For this review, take the finished solid that the model builds, in its own axes (mm). Give positions to 0.01 mm unless a question says otherwise; leave off trailing zeros. Write each loop counter-clockwise with the first axis right and the second up, starting at its lowest first coordinate (ties: lowest second). Pieces come first, ordered by that corner, then holes.
1) We need section A-A on x = 68. Give the boundary of the cut face in (y, z).
2) We need section C-C on x = 9. Give the boundary of the cut face in (y, z), and give its area (3 significant figures).
3) Wall thickness on line 1 along Y through (x, z) = (111, -2.2); line 2 along Y through (x, z) = (90, -2); line 3 along Y through (x, z) = (56, -2): over which ranges is each line inside the solid? List them lowest first.
4) For P1, Ø5, axis at x = 30, y = 98, coming from the -Z side, flat-tipped, find the tip position at first contact; note if it passes through.
5) We need section B-B on y = 22. Give the boundary of the cut face in (x, z), and give its area (3 significant figures).
Autodesk Inventor part; units mm, degrees
ref_plane "YZ Plane" through (0, 0, 0) normal (1, 0, 0) x (0, 1, 0)
ref_plane "XZ Plane" through (0, 0, 0) normal (0, 1, 0) x (-1, 0, 0)
ref_plane "XY Plane" through (0, 0, 0) normal (0, 0, 1) x (1, 0, 0)
sketch "Náčrt2" plane through (0, 0, 0) normal (0, 0, 1) x (1, 0, 0)
  line L0 (0, 0) -> (120, 0)
  line L1 (120, 0) -> (120, 120)
  line L2 (120, 120) -> (0, 120)
  line L3 (0, 120) -> (0, 0)
  circle A0 centre (34.5442, 85.4558) radius 2.5
  circle A1 centre (85.4558, 85.4558) radius 2.5
  circle A2 centre (34.5442, 34.5442) radius 2.5
  circle A3 centre (85.4558, 34.5442) radius 2.5
  circle A4 centre (40.5, 111) radius 2
  circle A5 centre (79.5, 111) radius 2
  circle A6 centre (9, 79.5) radius 2
  circle A7 centre (9, 40.5) radius 2
  circle A8 centre (111, 79.5) radius 2
  circle A9 centre (111, 40.5) radius 2
  circle A10 centre (79.5, 9) radius 2
  circle A11 centre (40.5, 9) radius 2
  circle A12 centre (30, 98) radius 2
  circle A13 centre (90, 98) radius 2
  circle A14 centre (90, 22) radius 2
  circle A15 centre (30, 22) radius 2
  line L4 (42.5, 82.5) -> (77.5, 82.5)
  line L5 (82.5, 77.5) -> (82.5, 42.5)
  line L6 (77.5, 37.5) -> (42.5, 37.5)
  line L7 (37.5, 42.5) -> (37.5, 77.5)
  arc A16 (37.5, 42.5) -> (42.5, 37.5) centre (42.5, 42.5) ccw
  arc A17 (77.5, 37.5) -> (82.5, 42.5) centre (77.5, 42.5) ccw
  arc A18 (42.5, 82.5) -> (37.5, 77.5) centre (42.5, 77.5) ccw
  arc A19 (82.5, 77.5) -> (77.5, 82.5) centre (77.5, 77.5) ccw
  point P0 (37.5, 82.5)
  point P1 (82.5, 37.5)
  point P2 (82.5, 82.5)
  point P3 (37.5, 37.5)
  dimension "d18" = 1
  dimension "d26" = 120
  dimension "d27" = 120
  dimension "d28" = 39
  dimension "d29" = 39
  dimension "d30" = 60
  dimension "d31" = 76
  dimension "d32" = 72
  dimension "d35" = 5
  dimension "d36" = 4
  dimension "d37" = 4
  dimension "d42" = 5
  dimension "d43" = 5
  dimension "d44" = 35
extrude "Vysunutí2" add sketch "Náčrt2" against normal blind 3
properties part number "Cougar_Base2"
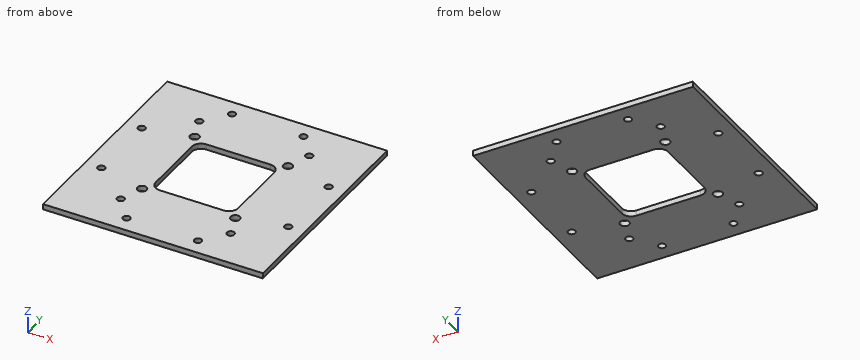
Results list:
1. outline: (0, -3) - (37.5, -3) - (37.5, 0) - (0, 0) - close; (82.5, -3) - (120, -3) - (120, 0) - (82.5, 0) - close
2. outline: (0, -3) - (38.5, -3) - (38.5, 0) - (0, 0) - close; (42.5, -3) - (77.5, -3) - (77.5, 0) - (42.5, 0) - close; (81.5, -3) - (120, -3) - (120, 0) - (81.5, 0) - close
2. area: 336 mm2
3. line 1: y = 0 to 38.5, 42.5 to 77.5, 81.5 to 120
3. line 2: y = 0 to 20, 24 to 96, 100 to 120
3. line 3: y = 0 to 37.5, 82.5 to 120
4. P1: stops at z = -3
5. outline: (0, -3) - (28, -3) - (28, 0) - (0, 0) - close; (32, -3) - (88, -3) - (88, 0) - (32, 0) - close; (92, -3) - (120, -3) - (120, 0) - (92, 0) - close
5. area: 336 mm2
